Design review of the part shown in the three views and the two pictorial views. Dimensions are in mm from the part's minimum x, y and z. A direction names the side the tool comes from. Give positions to 0.01 mm unless a question says otherwise; leave off trailing zeros. Order: outer loops, then holes, each group sorted by start corner. A loop starts at its lowest first (then second) coordinate and runs counter-clockwise, first axis right, second up.
Item 1: For P1, Ø5, axis at x = 54.5, z = 10.5, coming from the +Y side; P2, Ø2, axis at y = 26.5, z = 8.5, coming from the +X side; P3, Ø1, axis at x = 55.5, z = 10.5, coming from the -Y side; P4, Ø5, axis at x = 100.5, y = 39, coming from the -Z side, all flat-tipped, find the tip position at first contact; note any pin that passes through.
Item 2: The part is to be moulded in two halves that separate along Z. For the marked faces 5, 6 and 7, say which applies: released by +Z, released by -Z, zero draft, split by the parting line, or undercut.
Item 3: For probe 1 along X at (y, z) = (29.5, 3.25); probe 2 along X at (y, z) = (27, 13.25); probe 3 along X at (y, z) = (38.5, 5), list the stretches that pass through material, from the lowest coordinate up.
Item 4: Consider section A-A (y = 19). Give the boundary of the cut face in (x, z).
Item 5: Machinability: for the marked faces 1, 2, 3 and 4, which of the approach directions +Z, -Z, +X, -X, +Y, -Y give a long, thin tool a straight path to every point of the face, cutting with its end or side? Answer none if there is none.
Item 6: Consider section B-B (x = 49). Give the boundary of the cut face in (y, z), plus the area to 3 significant figures.
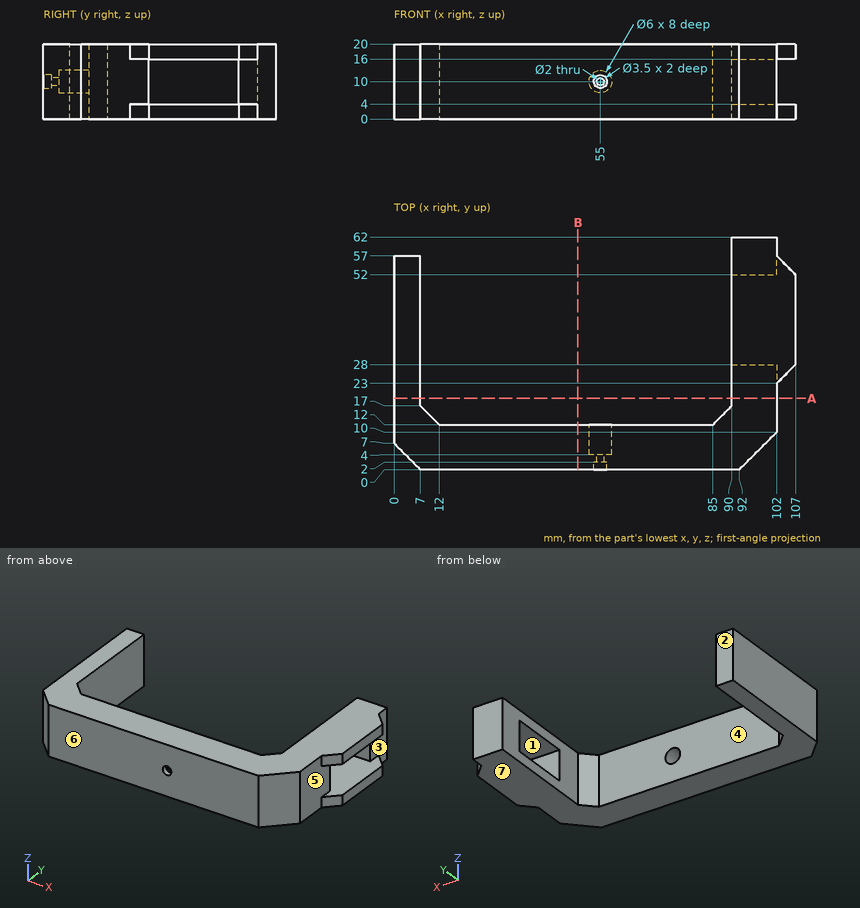
Resolved:
1. P1: stops at y = 12
1. P2: stops at x = 102
1. P3: stops at y = 2
1. P4: stops at z = 0
2. face 5: undercut
2. face 6: zero draft
2. face 7: released by -Z
3. probe 1: x = 0 to 7, 90 to 107
3. probe 2: x = 0 to 7, 90 to 102
3. probe 3: x = 0 to 7
4. outline: (0, 0) - (7, 0) - (7, 20) - (0, 20) - close; (90, 0) - (102, 0) - (102, 20) - (90, 20) - close
5. face 1: +X
5. face 2: +Z, -Z, -X, +Y
5. face 3: +X, +Y
5. face 4: +Z, -Z, +Y
6. outline: (0, 0) - (12, 0) - (12, 20) - (0, 20) - close
6. area: 240 mm2
